Geometry check sheet. Reference: the model listing, model coordinates, mm. A direction names the side the tool comes from. Round coordinates to 2 decimals unless told otherwise and drop trailing zeros. Order: outer loops, then holes, each group sorted by start corner. A loop starts at its lowest first (then second) coordinate and runs counter-clockwise, first axis right, second up. Notation, with made-up numbers: (6, 72.25) - (11, 72.25) arc R20 ccw to (11, 98.25) - close; hole circle Ø9 at (67, 57.25). An arc over 180 degrees is marked (long way). One line per question, with ' | ' between items. Start each with the question number.
Q1. Mould release check, pull along X, two halves, no side actions. Record for faces 4 (the face through (2.55, 0, 2)), 5 (the face through (0.172, 8.923, 0.246)), 6 (the face through (3, 0, 5)): +X half, -X half, draft (parallel to the pull), parting line (faces both ways), or undercut.
Q2. Material ranges on line 1 along Y through (x, z) = (2, 1.3); line 2 along Y through (x, z) = (-4.75, 2.5); line 3 along X through (y, z) = (-5.25, 3.9), recorded low to high.
Q3. Sectioned sample at A-A, the plane x = 2. Enter the section's corners in (y, z).
Q4. Tool access check on faces 1 (the face through (-6.68, 1.05, 2.48)), 2 (the face through (-3.95, 0, 1)), 3 (the face through (-9, -3.3, 0.5)). Record the directions out of +Z, -Z, +X, -X, +Y, -Y that give a thin tool (end or side, any length) a straight path to the whole face; none if there is none.
Q5. Sectioned sample at B-B, the plane y = 5.25. Enter the section's corners in (x, z).
Q6. Gauge pin test, flat ends, axial feed: P1, Ø2.5, axis at x = -2.5, z = 1.5, coming from the -Y side; P2, Ø1.2, axis at y = 1, z = 3.5, coming from the +X side; P3, Ø2.5, axis at y = -0.5, z = 2.5, coming from the -X side. Record the tip position at first contact, or that the pin passes through.
Q7. Sectioned sample at D-D, the plane z = 3.1. Enter the section's corners in (x, y).
Q8. Sectioned sample at C-C, the plane x = -7. Enter the section's corners in (y, z), then the cut area to 3 significant figures.
```python
from build123d import *

# Parameters (mm, degrees)
SKETCH1_R                   = 8.5
BOSS_EXTRUDE1_DEPTH         = 5
M2_HEXNUT_CUTOUT_DEPTH      = 1.4
M2_HEXNUT_CUTOUT_DEPTH_BACK = 1.4
SKETCH2_W                   = 5
SKETCH2_H                   = 4
FILLET1_R                   = 0.5
M2_THRU_DEPTH               = 16.111336804
SKETCH4_R                   = 9
SKETCH4_R_2                 = 8.5
BOSS_EXTRUDE2_DEPTH         = 0.5


with BuildPart() as part:
    # Sketch1 → Boss-Extrude1 (new body)
    with BuildSketch(Plane.XY):
        with Locations((-1, 0)):
            Circle(SKETCH1_R)
        Polygon((0, -2.944486373), (2.55, -1.472243186), (2.55, 1.472243186), (0, 2.944486373), (-2.55, 1.472243186), (-2.55, -1.472243186), align=None, mode=Mode.SUBTRACT)
    extrude(amount=BOSS_EXTRUDE1_DEPTH)

    # Sketch2 → M2 Hexnut Cutout (cut, two sides: drawn at the far end of the back side and taken through both)
    with BuildSketch(Plane(origin=(-2.55, 0, 0), x_dir=(0, 0, -1), z_dir=(1, 0, 0)).offset(-M2_HEXNUT_CUTOUT_DEPTH_BACK)):
        with Locations((-2.5, 0)):
            Rectangle(SKETCH2_W, SKETCH2_H)
    extrude(amount=M2_HEXNUT_CUTOUT_DEPTH + M2_HEXNUT_CUTOUT_DEPTH_BACK, mode=Mode.SUBTRACT)

    # Fillet1
    fillet1_edges = [part.edges().sort_by_distance(p)[0] for p in [
        (-1.635898385, 2, 2.5),
        (-1.635898385, -2, 2.5),
    ]]
    fillet(fillet1_edges, radius=FILLET1_R)

    # Sketch3 → M2 Thru (cut, through all)
    with BuildSketch(Plane(origin=(-3.95, 0, 0), x_dir=(0, 0, -1), z_dir=(1, 0, 0))):
        with BuildLine():
            Line((-3.7, 0), (-3.41875, -0.508329064))
            ThreePointArc((-3.41875, -0.508329064), (-2.5, -1.05), (-1.58125, -0.508329064))
            Line((-1.58125, -0.508329064), (-1.3, 0))
            Line((-1.3, 0), (-1.58125, 0.508329064))
            ThreePointArc((-1.58125, 0.508329064), (-2.5, 1.05), (-3.41875, 0.508329064))
            Line((-3.41875, 0.508329064), (-3.7, 0))
        make_face()
    extrude(amount=-M2_THRU_DEPTH, mode=Mode.SUBTRACT)

    # Sketch4 → Boss-Extrude2 (add)
    with BuildSketch(Plane(origin=(0, 0, 0), x_dir=(-1, 0, 0), z_dir=(0, 0, -1))):
        with Locations((1, 0)):
            Circle(SKETCH4_R)
        with Locations((1, 0)):
            Circle(SKETCH4_R_2, mode=Mode.SUBTRACT)
    extrude(amount=-BOSS_EXTRUDE2_DEPTH)


solid = part.part
```
Determined:
1) face 4: undercut | face 5: parting line | face 6: draft
2) line 1: y = -7.95 to -1.79, 1.79 to 7.95 | line 2: y = -7.63 to -1.05, 1.05 to 7.63 | line 3: x = -7.68 to 5.68
3) outline: (-8.49, 0) - (-1.79, 0) - (-1.79, 5) - (-7.95, 5) - (-7.95, 0.5) - (-8.49, 0.5) - close; (1.79, 0) - (8.49, 0) - (8.49, 0.5) - (7.95, 0.5) - (7.95, 5) - (1.79, 5) - close
4) face 1: -X | face 2: +Z, -Z | face 3: +Z
5) outline: (-8.31, 0) - (6.31, 0) - (6.31, 0.5) - (5.68, 0.5) - (5.68, 5) - (-7.68, 5) - (-7.68, 0.5) - (-8.31, 0.5) - close
6) P1: stops at y = -8.97 | P2: stops at x = 7.49 | P3: stops at x = -9.5
7) outline: (-9.46, -0.86) arc R8.5 ccw (long way) to (-9.46, 0.86) - (-3.95, 0.86) - (-3.95, 2) - (-1.77, 2) arc R0.5 ccw to (-1.52, 2.07) - (0, 2.94) - (2.55, 1.47) - (2.55, -1.47) - (0, -2.94) - (-1.52, -2.07) arc R0.5 ccw to (-1.77, -2) - (-3.95, -2) - (-3.95, -0.86) - close
8) outline: (-6.71, 0) - (6.71, 0) - (6.71, 0.5) - (6.02, 0.5) - (6.02, 5) - (-6.02, 5) - (-6.02, 0.5) - (-6.71, 0.5) - close; hole (-0.51, 1.58) - (0, 1.3) - (0.51, 1.58) arc R1.05 ccw to (0.51, 3.42) - (0, 3.7) - (-0.51, 3.42) arc R1.05 ccw to start | area: 57.3 mm2
